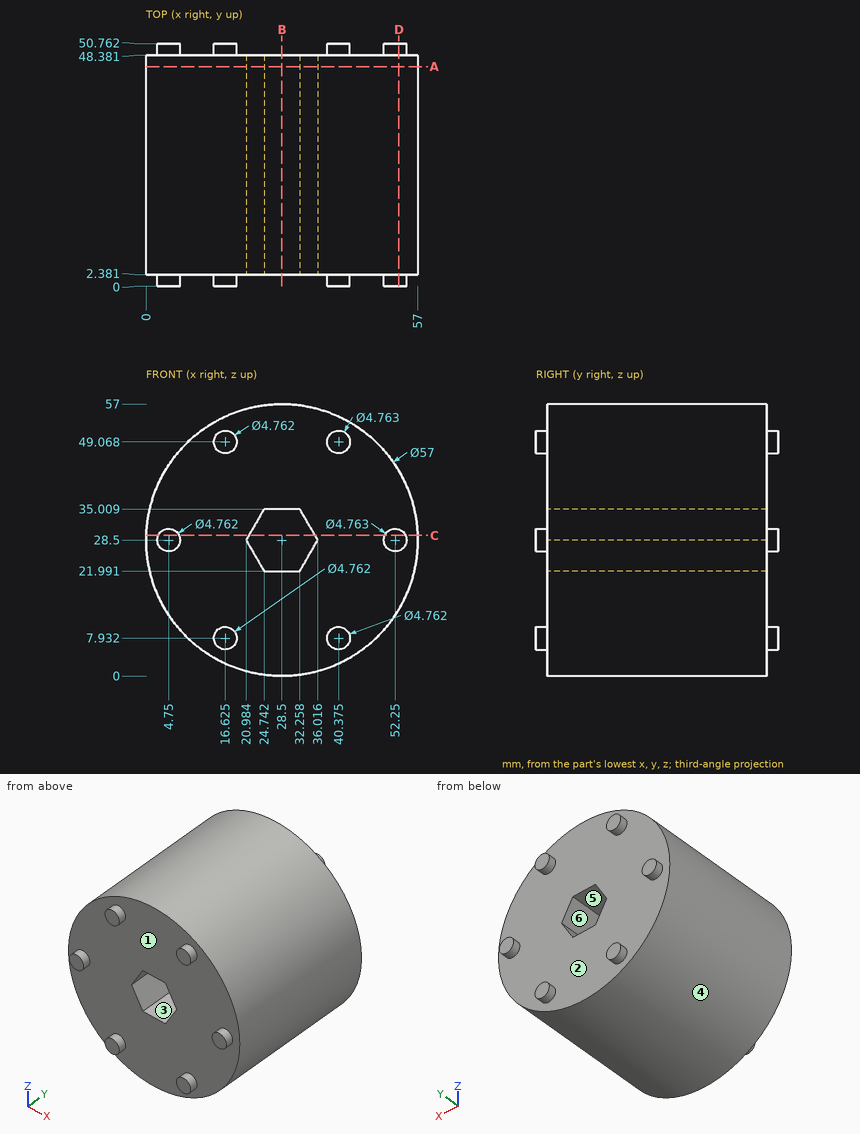
Could you check a few things on this drawing? It's one solid part, dimensions in mm from its lowest x, y, z. A direction names the side the tool comes from. Give positions to 0.01 mm unless a question says otherwise; leave off trailing zeros. Order: outer loops, then holes, each group sorted by start corner. A loop starts at its lowest first (then second) coordinate and runs counter-clockwise, first axis right, second up. Notation, with made-up numbers: (65.25, 78) - (99.25, 78) arc R15 ccw to (99.25, 104) - close; hole circle Ø8 at (-31.5, 65). An arc over 180 degrees is marked (long way). One line per question, with ' | ' between items. Start each with the question number.
Item 1: I want a section at A-A on y = 46. Write out the boundary of the cut face in (x, z) (1 decimal), then the cut area to 4 significant figures.
Item 2: For the marked faces 1, 2 and 3, which set-ups out of +Z, -Z, +X, -X, +Y, -Y let a thin tool reach every point of the face, with its end or its side?
Item 3: I need wall thicknesses on probe 1 along Y at (x, z) = (21.5, 21); probe 2 along Z at (x, y) = (32, 28.5) (1 decimal); probe 3 along X at (y, z) = (29.5, 33). Which ranges of each line are inside material? Lowest first, please. Write a range as [from, to].
Item 4: I'm going to push flat-ended pins straight in: pin 1 Ø4 at (x, z) = (10.5, 6) entering from -Y; pin 2 Ø8 at (x, y) = (10, 5.5) entering from +Z (1 decimal); pin 3 Ø1 at (y, z) = (8.5, 32) entering from +X. Where does each tip first touch, or does it pass through?
Item 5: I want a section at B-B on x = 28.5. Write out the boundary of the cut face in (y, z), then the cut area to 3 significant figures.
Item 6: Thinking about a two-plate mould opening in X: for the marked faces 4, 5 and 6, which applies, pulls with the +X half, pulls with the -X half, needs draft (parallel to the pull), parting line crosses it, or undercut?
Item 7: I want a section at C-C on z = 29.5. Write out the boundary of the cut face in (x, y), then the cut area to 3 significant figures.
Item 8: I want a section at D-D on x = 53. Write out the boundary of the cut face in (y, z), then the cut area to 3 significant figures.
Verdict:
1) outline: circle Ø57 at (28.5, 28.5); hole (21, 28.5) - (24.7, 22) - (32.3, 22) - (36, 28.5) - (32.3, 35) - (24.7, 35) - close | area: 2,405 mm^2
2) face 1: -Y | face 2: +Y | face 3: +Y, -Y
3) probe 1: [2.38, 48.38] | probe 2: [0.2, 22], [35, 56.8] | probe 3: [0.36, 23.58], [33.42, 56.64]
4) pin 1: y = 2.38 | pin 2: z = 53 | pin 3: x = 56.84
5) outline: (2.38, 0) - (48.38, 0) - (48.38, 21.99) - (2.38, 21.99) - close; (2.38, 35.01) - (48.38, 35.01) - (48.38, 57) - (2.38, 57) - close | area: 2,020 mm^2
6) face 4: parting line crosses it | face 5: undercut | face 6: undercut
7) outline: (0.02, 2.38) - (2.59, 2.38) - (2.59, 0) - (6.91, 0) - (6.91, 2.38) - (21.56, 2.38) - (21.56, 48.38) - (6.91, 48.38) - (6.91, 50.76) - (2.59, 50.76) - (2.59, 48.38) - (0.02, 48.38) - close; (35.44, 2.38) - (50.09, 2.38) - (50.09, 0) - (54.41, 0) - (54.41, 2.38) - (56.98, 2.38) - (56.98, 48.38) - (54.41, 48.38) - (54.41, 50.76) - (50.09, 50.76) - (50.09, 48.38) - (35.44, 48.38) - close | area: 2,020 mm^2
8) outline: (0, 26.24) - (2.38, 26.24) - (2.38, 13.94) - (48.38, 13.94) - (48.38, 26.24) - (50.76, 26.24) - (50.76, 30.76) - (48.38, 30.76) - (48.38, 43.06) - (2.38, 43.06) - (2.38, 30.76) - (0, 30.76) - close | area: 1,360 mm^2
